Source: three-view drawing plus pictorial views. Frame: mm from the lowest corner of the part. A direction names the side the tool comes from. Give positions to 0.01 mm unless a question says otherwise; leave off trailing zeros. Order: outer loops, then holes, each group sorted by start corner. A loop starts at its lowest first (then second) coordinate and runs counter-clockwise, first axis right, second up. Notation, with made-up numbers: (-24.75, 35) - (-6.75, 35) arc R9 ccw to (-6.75, 44) - close; hole circle Ø11 at (80, -7). An arc over 180 degrees is marked (long way). Use CSV: the item, a comma, the result in double quotes.
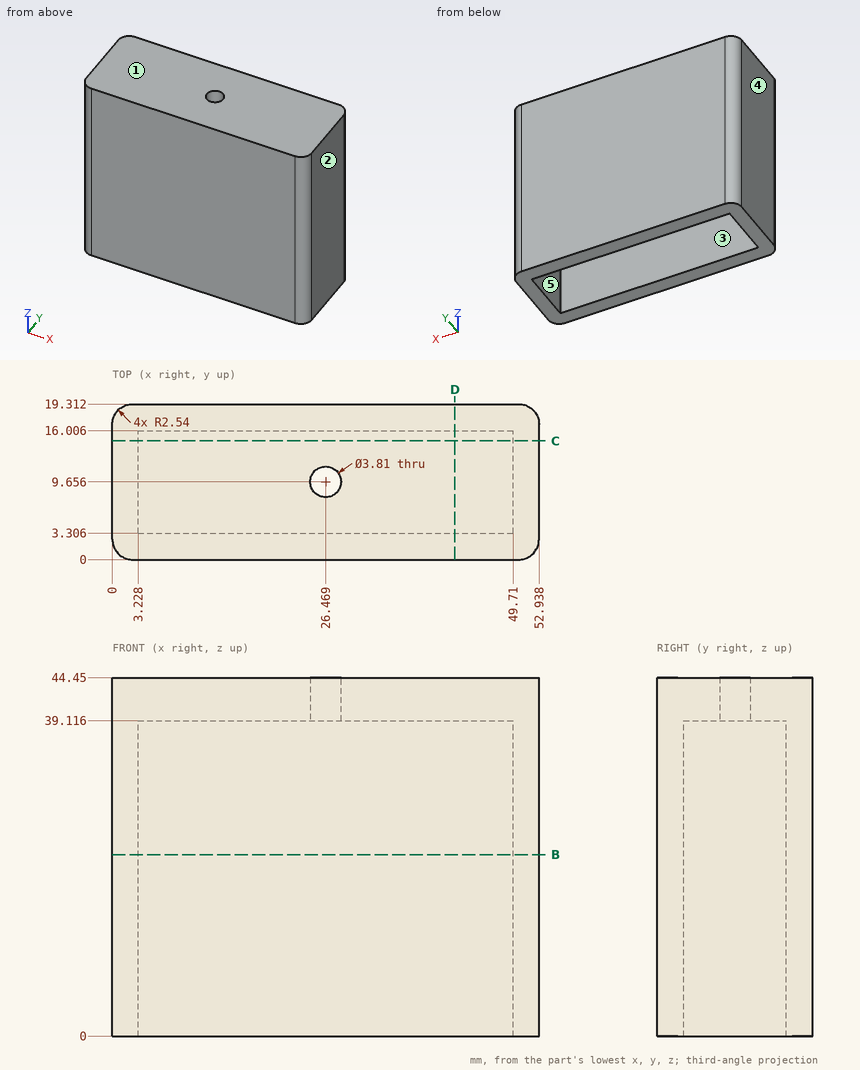
Item 1: First-contact query: pin 1 (6 mm diameter, centred on x = 26.47, y = 9.66, fed in from -Z). Flat tip, straight axial feed; report the tip coordinate or a pass-through.
Filled in:
pin 1,"stops at z = 39.12"
Item 2: Section B-B on z = 22.5. Return the cut outline in (x, y).
Filled in:
outline,"(0, 2.54) arc R2.54 ccw to (2.54, 0) - (50.4, 0) arc R2.54 ccw to (52.94, 2.54) - (52.94, 16.77) arc R2.54 ccw to (50.4, 19.31) - (2.54, 19.31) arc R2.54 ccw to (0, 16.77) - close; hole (3.23, 3.31) - (49.71, 3.31) - (49.71, 16.01) - (3.23, 16.01) - close"
Item 3: Section D-D on x = 42.5. Return the cut outline in (y, z).
Filled in:
outline,"(0, 0) - (3.31, 0) - (3.31, 39.12) - (16.01, 39.12) - (16.01, 0) - (19.31, 0) - (19.31, 44.45) - (0, 44.45) - close"
Item 4: Material intervals for line 1 (Y direction, x = 15.5, z = 20.5); line 2 (X direction, y = 7.5, z = 7); line 3 (Z direction, x = 44, y = 13.5), sorted ascending. Write a range as from..to.
Filled in:
line 1,"y = 0..3.31, 16.01..19.31"
line 2,"x = 0..3.23, 49.71..52.94"
line 3,"z = 39.12..44.45"
Item 5: Mould query, pull axis X, two halves, no side actions, for the marked faces 1, 2 and 3. Classes: released by +X, released by -X, zero draft, split by the parting line, or undercut.
Filled in:
face 1,"zero draft"
face 2,"released by +X"
face 3,"undercut"
Item 6: Section C-C on y = 14.75. Return the cut outline in (x, z), then the cut area to 3 significant figures.
Filled in:
outline,"(0, 0) - (3.23, 0) - (3.23, 39.12) - (49.71, 39.12) - (49.71, 0) - (52.94, 0) - (52.94, 44.45) - (0, 44.45) - close"
area,"535 mm2"
Item 7: Set-up query: the marked faces 4 and 5. Return all of +Z, -Z, +X, -X, +Y, -Y with unobstructed straight access to the full face (end or side cutting, diameter ignored); none if empty.
Filled in:
face 4,"+Z, -Z, -X, +Y, -Y"
face 5,"-Z"
